Can you work these out from the model? Positions are in its coordinate system, mm. A direction names the side the tool comes from. Give positions to 0.01 mm unless a question says otherwise; leave off trailing zeros. Loops run counter-clockwise (first coordinate to the right, second up) from the corner with the lowest first, then second, coordinate; pieces in that order, holes last. Notation, with made-up numbers: M -1,-17 L 10,-17 A29 ccw 10,17 Z; hole C -35,66.5 d8. An arc over 180 degrees is marked long. Put each result on its own line as item: value. Start each with the question number.
1) Imagine slicing it at A-A (y = 28.4). Write out the boundary of the cut face in (x, z).
2) For faces 1 (the cylindrical face through (10.86, 29.93, -9.77)), 2 (the flat face through (19, 27, -11.75)), which set-ups out of +Z, -Z, +X, -X, +Y, -Y let a thin tool reach every point of the face, with its end or its side?
3) If we mould it in two halves opening along X, with no side actions, what happens to faces 3 (the flat face through (35.27, 27, -8)), 4 (the flat face through (10.874, 28.887, -9.697)), 5 (the cylindrical face through (3.18, 27.41, -4.7))? For each: +X half, -X half, draft (parallel to the pull), parting line (faces both ways), or undercut.
4) Please list where these lines run through material, in increasing order: line 1 along Z through (x, y) = (16.5, 29.65); line 2 along Y through (x, z) = (11, -7.5); line 3 along Z through (x, y) = (14, 29.65). Write a range as from..to.
from build123d import *

# Parameters (mm, degrees)
PAD001_DEPTH            = 10
BODY001_PLACEMENT_ANGLE = 90
PAD003_DEPTH            = 10
BODY003_PLACEMENT_ANGLE = 270
BOX005_W                = 32.52
BOX005_H                = 5
BOX005_DEPTH            = 7.5
FILLET002_R             = 1.5
FILLET003_R             = 0.25


with BuildPart() as body001:
    # Sketch001 → Pad001 (new body)
    with BuildSketch(Plane.XZ):
        with BuildLine():
            Line((-0.253994, 6.623128), (-3.180974, -6.757813))
            ThreePointArc((-3.180974, -6.757813), (-3.12952, -6.976398), (-2.926979, -7.073373))
            Line((-2.926979, -7.073373), (2.926979, -7.073373))
            ThreePointArc((2.926979, -7.073373), (3.12952, -6.976398), (3.180974, -6.757813))
            Line((3.180974, -6.757813), (0.253994, 6.623128))
            ThreePointArc((0.253994, 6.623128), (0, 6.827569), (-0.253994, 6.623128))
        make_face()
    extrude(amount=PAD001_DEPTH)


with BuildPart() as body001_1:
    # Body001 placement: moved
    add(body001.part.moved(Location((27.1, 63, -8))).rotate(Axis((27.1, 63, -8), (0, 1, 0)), BODY001_PLACEMENT_ANGLE))


with BuildPart() as wedge_holes:
    # Sketch003 → Pad003 (new body)
    with BuildSketch(Plane.XZ):
        with BuildLine():
            Line((-0.253994, 6.623128), (-3.180974, -6.757813))
            ThreePointArc((-3.180974, -6.757813), (-3.12952, -6.976398), (-2.926979, -7.073373))
            Line((-2.926979, -7.073373), (2.926979, -7.073373))
            ThreePointArc((2.926979, -7.073373), (3.12952, -6.976398), (3.180974, -6.757813))
            Line((3.180974, -6.757813), (0.253994, 6.623128))
            ThreePointArc((0.253994, 6.623128), (0, 6.827569), (-0.253994, 6.623128))
        make_face()
    extrude(amount=PAD003_DEPTH)


with BuildPart() as wedge_holes_1:
    # Body003 placement: moved
    add(wedge_holes.part.moved(Location((10.9, 63, -8))).rotate(Axis((10.9, 63, -8), (0, 1, 0)), BODY003_PLACEMENT_ANGLE))

    # Fusion003: union Body001
    add(body001_1.part)


with BuildPart() as wedge_holes_2:
    # Fusion003 placement: moved
    add(wedge_holes_1.part.moved(Location((0, -25, 0))))


with BuildPart() as fillet003:
    # Box005 → Box005 (new body)
    with BuildSketch(Plane(origin=(2.75, 25, -11.75), x_dir=(1, 0, 0), z_dir=(0, 0, 1))):
        with Locations((16.26, 2.5)):
            Rectangle(BOX005_W, BOX005_H)
    extrude(amount=BOX005_DEPTH)

    # Fillet002
    fillet002_edges = [fillet003.edges().sort_by_distance(p)[0] for p in [
        (2.75, 27.5, -4.25),
        (2.75, 27.5, -11.75),
        (35.27, 27.5, -4.25),
        (35.27, 27.5, -11.75),
    ]]
    fillet(fillet002_edges, radius=FILLET002_R)

    # Cut003: cut wedge holes
    add(wedge_holes_2.part, mode=Mode.SUBTRACT)

    # Fillet003
    fillet003_edges = [fillet003.edges().sort_by_distance(p)[0] for p in [
        (2.75, 30, -8),
        (3.18934, 30, -11.31066),
        (19.01, 30, -11.75),
        (34.83066, 30, -11.31066),
        (35.27, 30, -8),
        (3.18934, 30, -4.68934),
        (34.83066, 30, -4.68934),
        (19.01, 30, -4.25),
        (4.072431, 30, -8),
        (10.967343, 30, -6.282516),
        (17.876398, 30, -4.87048),
        (17.973373, 30, -8),
        (17.876398, 30, -11.12952),
        (10.967343, 30, -9.717484),
        (33.927569, 30, -8),
        (27.032657, 30, -9.717484),
        (20.123602, 30, -11.12952),
        (20.026627, 30, -8),
        (20.123602, 30, -4.87048),
        (27.032657, 30, -6.282516),
    ]]
    fillet(fillet003_edges, radius=FILLET003_R)


solid = fillet003.part
Recorded:
1. outline: M 2.75,-10.25 A1.5 ccw 4.25,-11.75 L 33.77,-11.75 A1.5 ccw 35.27,-10.25 L 35.27,-5.75 A1.5 ccw 33.77,-4.25 L 4.25,-4.25 A1.5 ccw 2.75,-5.75 Z; hole M 4.28,-8.25 L 17.66,-11.18 A0.26 ccw 17.97,-10.93 L 17.97,-5.07 A0.26 ccw 17.66,-4.82 L 4.28,-7.75 A0.26 ccw Z; hole M 20.03,-10.93 A0.26 ccw 20.34,-11.18 L 33.72,-8.25 A0.26 ccw 33.72,-7.75 L 20.34,-4.82 A0.26 ccw 20.03,-5.07 Z
2. face 1: +Y
2. face 2: -Z, +X, -X, +Y, -Y
3. face 3: +X half
3. face 4: undercut
3. face 5: -X half
4. line 1: -11.75..-10.93, -5.07..-4.25
4. line 2: 25..28
4. line 3: -11.75..-10.38, -5.62..-4.25
